Build history of the part. All positions in model axes, mm. A direction names the side the tool comes from. Give positions to 0.01 mm unless a question says otherwise; leave off trailing zeros. Order: outer loops, then holes, each group sorted by start corner. A loop starts at its lowest first (then second) coordinate and runs counter-clockwise, first axis right, second up. Notation, with made-up numbers: (-39, 45.25) - (-18, 45.25) arc R21 ccw to (-18, 64.25) - close; hole circle Ø5 at (28.25, -30.5). An arc over 180 degrees is marked (long way). Use a Markdown table: item, result.
from build123d import *
from OCP.BRepFilletAPI import BRepFilletAPI_MakeChamfer

# Parameters (mm, degrees)
SKETCH1_R           = 10
BOSS_EXTRUDE1_DEPTH = 28.5
BOSS_EXTRUDE2_DEPTH = 45
CUT_EXTRUDE1_DEPTH  = 30
CIRPATTERN1_COUNT   = 2
CHAMFER1_SIZE       = 50
CHAMFER1_SIZE2      = 13.397459622
FILLET3_R           = 15
CHAMFER2_SIZE       = 90
CHAMFER2_SIZE2      = 13.607292824
CUT_EXTRUDE2_DEPTH  = 138.142132616
CUT_EXTRUDE4_DEPTH  = 22.15
FILLET6_R           = 6.35


with BuildPart() as part:
    # Sketch1 → Boss-Extrude1 (new body)
    with BuildSketch(Plane.XY):
        Polygon((-7.047570808, -123.427136592), (39.353608362, 123.427136592), (7.047570808, 123.427136592), (-39.353608362, -123.427136592), align=None)
        with Locations(Location((0, 0, 0), (0, 0, 180))):
            Circle(SKETCH1_R, mode=Mode.SUBTRACT)
    extrude(amount=BOSS_EXTRUDE1_DEPTH)

    # Sketch2 → Boss-Extrude2 (add)
    with BuildSketch(Plane(origin=(0, 0, 0), x_dir=(-1, 0, 0), z_dir=(0, 0, -1))):
        Polygon((-39.353608362, 123.427136592), (-36.488946708, 108.187136592), (-4.182909154, 108.187136592), (-7.047570808, 123.427136592), align=None)
        Polygon((36.488946708, -108.187136592), (4.182909154, -108.187136592), (7.047570808, -123.427136592), (39.353608362, -123.427136592), align=None)
    extrude(amount=BOSS_EXTRUDE2_DEPTH)

    # Sketch4 → Cut-Extrude1 (cut)
    with BuildSketch(Plane(origin=(0, 123.427136592, 0), x_dir=(1, 0, 0), z_dir=(0, 1, 0))):
        with BuildLine():
            ThreePointArc((18.438089585, 30.433032299), (19.83299354, 27.065436254), (23.200589585, 25.670532299))
            Line((23.200589585, 25.670532299), (23.200589585, 30.433032299))
            Line((23.200589585, 30.433032299), (18.438089585, 30.433032299))
        make_face()
        with BuildLine():
            Line((23.200589585, 30.433032299), (23.200589585, 25.670532299))
            ThreePointArc((23.200589585, 25.670532299), (26.56818563, 27.065436254), (27.963089585, 30.433032299))
            Line((27.963089585, 30.433032299), (23.200589585, 30.433032299))
        make_face()
        with BuildLine():
            Line((18.438089585, 30.433032299), (23.200589585, 30.433032299))
            Line((23.200589585, 30.433032299), (23.200589585, 35.195532299))
            ThreePointArc((23.200589585, 35.195532299), (19.83299354, 33.800628344), (18.438089585, 30.433032299))
        make_face()
        with BuildLine():
            Line((23.200589585, 35.195532299), (23.200589585, 30.433032299))
            Line((23.200589585, 30.433032299), (27.963089585, 30.433032299))
            ThreePointArc((27.963089585, 30.433032299), (26.56818563, 33.800628344), (23.200589585, 35.195532299))
        make_face()
    cut_extrude1 = extrude(amount=-CUT_EXTRUDE1_DEPTH, mode=Mode.SUBTRACT)

    # CirPattern1: Cut-Extrude1 ×2 about axis
    cirpattern1_axis = Axis((0, 0, 28.5), (0, 0, -1))
    for i in range(1, CIRPATTERN1_COUNT):
        add(cut_extrude1.rotate(cirpattern1_axis, i * 360 / CIRPATTERN1_COUNT), mode=Mode.SUBTRACT)

    # Chamfer1: one chamfer whose edges measure the first distance from different faces: ONE call of the kernel's chamfer builder (chamfer() names one face for all edges)
    chamfer1_edges_1 = [part.edges().sort_by_distance(p)[0] for p in [
        (-23.200589585, -123.427136592, 28.5),
    ]]
    chamfer1_side_1 = [part.faces().sort_by_distance(p)[0] for p in [
        (-23.200589585, -123.427136592, -7.563719055),
    ]]
    chamfer1_edges_2 = [part.edges().sort_by_distance(p)[0] for p in [
        (23.200589585, 123.427136592, 28.5),
    ]]
    chamfer1_side_2 = [part.faces().sort_by_distance(p)[0] for p in [
        (23.200589585, 123.427136592, -7.563719055),
    ]]
    chamfer1 = BRepFilletAPI_MakeChamfer(part.part.solid().wrapped)
    for e in chamfer1_edges_1:
        chamfer1.Add(CHAMFER1_SIZE, CHAMFER1_SIZE2, e.wrapped, chamfer1_side_1[0].wrapped)  # the first distance lies on this face
    for e in chamfer1_edges_2:
        chamfer1.Add(CHAMFER1_SIZE, CHAMFER1_SIZE2, e.wrapped, chamfer1_side_2[0].wrapped)  # the first distance lies on this face
    add(Compound.cast(chamfer1.Shape()), mode=Mode.REPLACE)

    # Fillet3
    fillet3_edges = [part.edges().sort_by_distance(p)[0] for p in [
        (20.335927931, 108.187136592, 0),
        (-20.335927931, -108.187136592, 0),
    ]]
    fillet(fillet3_edges, radius=FILLET3_R)

    # Chamfer2
    chamfer2_edges = [part.edges().sort_by_distance(p)[0] for p in [
        (-20.682270107, -110.02967697, 28.5),
        (20.682270107, 110.02967697, 28.5),
    ]]
    chamfer2_side = [part.faces().sort_by_distance(p)[0] for p in [
        (13.872325433, 0.428701757, 28.5),
    ]]
    chamfer(chamfer2_edges, length=CHAMFER2_SIZE, length2=CHAMFER2_SIZE2, reference=chamfer2_side[0])

    # Sketch10 → Cut-Extrude2 (cut, symmetric)
    with BuildSketch(Plane(origin=(0, 0, 0), x_dir=(0, 0, -1), z_dir=(1, 0, 0))):
        with BuildLine():
            Line((-28.5, 20.02967697), (-11.939027322, 98.847487856))
            ThreePointArc((-11.939027322, 98.847487856), (-4.989688501, 112.112334692), (7.875417438, 119.776440697))
            Line((7.875417438, 119.776440697), (-24.698068362, 128.387749722))
            Line((-24.698068362, 128.387749722), (-33.956814005, 23.522391457))
            Line((-33.956814005, 23.522391457), (-28.5, 20.02967697))
        make_face()
    cut_extrude2 = extrude(amount=CUT_EXTRUDE2_DEPTH, both=True, mode=Mode.SUBTRACT)

    # Mirror1: Cut-Extrude2 across plane
    add(cut_extrude2.mirror(Plane.ZX), mode=Mode.SUBTRACT)

    # Sketch11 → Cut-Extrude4 (cut)
    with BuildSketch(Plane.XY.offset(28.5)):
        Polygon((14.650397163, 26.37967697), (-4.73322537, 26.37967697), (7.694934571, 92.497487856), (27.078557104, 92.497487856), align=None)
        Polygon((-14.650397163, -26.37967697), (4.73322537, -26.37967697), (-7.694934571, -92.497487856), (-27.078557104, -92.497487856), align=None)
    extrude(amount=-CUT_EXTRUDE4_DEPTH, mode=Mode.SUBTRACT)

    # Fillet6
    fillet6_edges = [part.edges().sort_by_distance(p)[0] for p in [
        (14.650397163, 26.37967697, 16.757878094),
        (-4.73322537, 26.37967697, 16.757878094),
        (7.694934571, 92.497487856, 9.811635567),
        (27.078557104, 92.497487856, 9.811635567),
        (-27.078557104, -92.497487856, 9.811635567),
        (-7.694934571, -92.497487856, 9.811635567),
        (4.73322537, -26.37967697, 16.757878094),
        (-14.650397163, -26.37967697, 16.757878094),
    ]]
    fillet(fillet6_edges, radius=FILLET6_R)


solid = part.part
1) Tool access for faces 3 (the flat face through (-21, -108.187, -26)), 4 (the flat face through (-11, -59, 6.35)), 5 (the flat face through (-21.314, -58.887, 20.335)): list every direction of +Z, -Z, +X, -X, +Y, -Y with a clear straight run to the whole face (end or side of a thin tool).
Computed:
| item | result |
|---|---|
| face 3 | -Z, +X, -X, +Y |
| face 4 | +Z |
| face 5 | +Z, +X, -X, -Y |
2) Slice it at C-C (y = -80). Write the cut outline in (x, z).
Computed:
| item | result |
|---|---|
| outline | (-31.19, 0) - (1.12, 0) - (1.12, 15.9) - (-5.35, 15.9) - (-5.35, 6.35) - (-24.73, 6.35) - (-24.73, 15.9) - (-31.19, 15.9) - close |
3) Slice it at B-B (z = 18.5). Write the cut outline in (x, y), and give its area (3 significant figures).
Computed:
| item | result |
|---|---|
| outline | (-28.86, -67.62) - (-22.4, -67.62) - (-15.62, -31.56) arc R6.35 cw to (-9.38, -26.38) - (-2.92, -26.38) arc R6.35 cw to (3.32, -33.9) - (-3.02, -67.62) - (3.44, -67.62) - (28.86, 67.62) - (22.4, 67.62) - (15.62, 31.56) arc R6.35 cw to (9.38, 26.38) - (2.92, 26.38) arc R6.35 cw to (-3.32, 33.9) - (3.02, 67.62) - (-3.44, 67.62) - close; hole circle Ø20 at (0, 0) |
| area | 2,490 mm² |
4) Slice it at A-A (z = -40). Write the cut outline in (x, y), and give its area (3 significant figures).
Computed:
| item | result |
|---|---|
| outline | (-39.35, -123.43) - (-7.05, -123.43) - (-4.18, -108.19) - (-36.49, -108.19) - close; (4.18, 108.19) - (36.49, 108.19) - (39.35, 123.43) - (7.05, 123.43) - close |
| area | 985 mm² |
5) Wall check: line 1 (Y direction, x = -34.5, z = -27); line 2 (Y direction, x = 12, z = -39.5); line 3 (X direction, y = -59, z = 13.5). Give the ranges that are in metal, low to high. Write a range as from..to.
Computed:
| item | result |
|---|---|
| line 1 | y = -123.43..-108.19 |
| line 2 | y = 108.19..123.43 |
| line 3 | x = -27.24..-20.78, -1.4..5.06 |
6) Two-plate mould, pull along X, no slides. Class faces 1 (the cylindrical face through (10, 0, 14)), 2 (the flat face through (23, 123.427, -36)): +X half, -X half, draft (parallel to the pull), parting line (faces both ways), or undercut.
Computed:
| item | result |
|---|---|
| face 1 | undercut |
| face 2 | draft |
7) Slice it at D-D (x = 31). Write the cut outline in (y, z).
Computed:
| item | result |
|---|---|
| outline | (78.99, 0) - (93.19, 0) arc R15 cw to (108.19, -15) - (108.19, -45) - (123.43, -45) - (123.43, -21.5) - (119.78, -7.88) arc R27.53 ccw to (98.85, 11.94) - (78.99, 16.11) - close |
8) Pin check, flat tips, straight feed: P1, Ø7, axis at x = -5.5, z = 12.5, coming from the -Y side; P2, Ø24, axis at x = 22.5, z = -27, coming from the -Y side; P3, Ø8, axis at x = -19, z = -29, coming from the +Y side. Stop position of each tip, or through.
Computed:
| item | result |
|---|---|
| P1 | stops at y = -106.67 |
| P2 | stops at y = 108.19 |
| P3 | stops at y = -108.19 |
